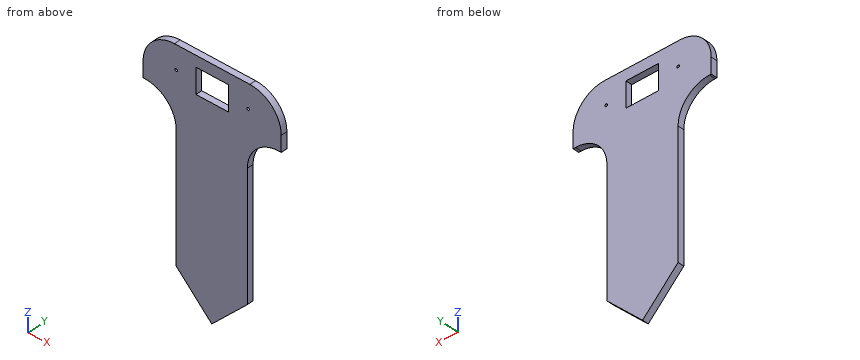
from build123d import *

# Parameters (mm, degrees)
SKETCH2_W               = 44
SKETCH2_H               = 15
BOSS_EXTRUDE1_DEPTH     = 2
SKETCH3_W               = 10.3
SKETCH3_H               = 8
CUT_EXTRUDE1_DEPTH      = 2
SKETCH5_R               = 0.4
CUT_EXTRUDE2_DEPTH      = 2
SKETCH6_W               = 22.666596939
SKETCH6_H               = 61.385041888
BOSS_EXTRUDE3_DEPTH     = 2
FILLET1_R               = 10
CUT_EXTRUDE3_DEPTH      = 73.340507297
CUT_EXTRUDE3_DEPTH_BACK = 2
CUT_EXTRUDE4_DEPTH      = 73.340507297
CUT_EXTRUDE4_DEPTH_BACK = 2
FILLET2_R               = 10


with BuildPart() as part:
    # Sketch2 → Boss-Extrude1 (new body)
    with BuildSketch(Plane(origin=(0, 0, 0), x_dir=(1, 0, 0), z_dir=(0, 1, 0))):
        Rectangle(SKETCH2_W, SKETCH2_H)
    extrude(amount=BOSS_EXTRUDE1_DEPTH)

    # Sketch3 → Cut-Extrude1 (cut)
    with BuildSketch(Plane(origin=(0, 2, 0), x_dir=(1, 0, 0), z_dir=(0, 1, 0))):
        Rectangle(SKETCH3_W, SKETCH3_H)
    extrude(amount=-CUT_EXTRUDE1_DEPTH, mode=Mode.SUBTRACT)

    # Sketch5 → Cut-Extrude2 (cut)
    with BuildSketch(Plane(origin=(0, 2, 0), x_dir=(1, 0, 0), z_dir=(0, 1, 0))):
        with Locations(Location((-11.45, 0, 0), (0, 0, 270))):
            Circle(SKETCH5_R)
    cut_extrude2 = extrude(amount=-CUT_EXTRUDE2_DEPTH, mode=Mode.SUBTRACT)

    # Mirror1: Cut-Extrude2 across plane
    add(cut_extrude2.mirror(Plane(origin=(0, 0, 0), x_dir=(0, 0, 1), z_dir=(1, 0, 0))), mode=Mode.SUBTRACT)

    # Sketch6 → Boss-Extrude3 (add)
    with BuildSketch(Plane(origin=(0, 2, 0), x_dir=(1, 0, 0), z_dir=(0, 1, 0))):
        with Locations((-0.116701531, 38.192520944)):
            Rectangle(SKETCH6_W, SKETCH6_H)
    extrude(amount=-BOSS_EXTRUDE3_DEPTH)

    # Fillet1
    fillet1_edges = [part.edges().sort_by_distance(p)[0] for p in [
        (-11.45, 1, -7.5),
        (11.216596939, 1, -7.5),
    ]]
    fillet(fillet1_edges, radius=FILLET1_R)

    # Sketch8 → Cut-Extrude3 (cut, two sides: drawn at the far end of the back side and taken through both)
    with BuildSketch(Plane(origin=(0, 2, 0), x_dir=(1, 0, 0), z_dir=(0, 1, 0)).offset(-CUT_EXTRUDE3_DEPTH_BACK)):
        Polygon((119.416120766, 188.417864185), (-0.11670153, 68.885041888), (-11.45, 57.551743419), (-130.982822296, -61.981078878), (-370.048466889, 177.084565715), (-119.649523827, 427.483508777), align=None)
    extrude(amount=CUT_EXTRUDE3_DEPTH + CUT_EXTRUDE3_DEPTH_BACK, mode=Mode.SUBTRACT)

    # Sketch9 → Cut-Extrude4 (cut, two sides: drawn at the far end of the back side and taken through both)
    with BuildSketch(Plane(origin=(0, 2, 0), x_dir=(1, 0, 0), z_dir=(0, 1, 0)).offset(-CUT_EXTRUDE4_DEPTH_BACK)):
        Polygon((-119.649523827, 188.417864185), (-0.11670153, 68.885041888), (11.216596939, 57.551743419), (130.749419236, -61.981078878), (369.815063828, 177.084565715), (119.416120766, 427.483508777), align=None)
    extrude(amount=CUT_EXTRUDE4_DEPTH + CUT_EXTRUDE4_DEPTH_BACK, mode=Mode.SUBTRACT)

    # Fillet2
    fillet2_edges = [part.edges().sort_by_distance(p)[0] for p in [
        (22, 1, 7.5),
        (-22, 1, 7.5),
    ]]
    fillet(fillet2_edges, radius=FILLET2_R)


solid = part.part
Build history of the part. All positions in model axes, mm. Round coordinates to 2 decimals unless told otherwise and drop trailing zeros. Write each loop counter-clockwise with the first axis right and the second up, starting at its lowest first coordinate (ties: lowest second). Pieces come first, ordered by that corner, then holes. Notation, with made-up numbers: (-26.75, 49) -> (25.25, 49) arc R30 cw to (25.25, 84) -> close; hole circle Ø2 at (44, 14). An arc over 180 degrees is marked (long way). Use one line per item in the form item = value.
Q1. Drill centre lines: L1, parallel to X at y = 1.2, z = -42.5; L2, parallel to X at y = 0.4, z = 0; L3, parallel to Z at x = -4.5, y = 1.25. Where is each one in solid material? Low to high.
Conclusion:
L1 = -11.45 to 11.22
L2 = -21.68 to -11.85, -11.05 to -5.15, 5.15 to 11.05, 11.85 to 21.68
L3 = -64.5 to -4, 4 to 7.5
Q2. Band-saw the part on C-C, the plane x = 1.5. Write the cut outline in (y, z), then the cut area to 3 significant figures.
Conclusion:
outline = (0, -67.27) -> (2, -67.27) -> (2, -4) -> (0, -4) -> close; (0, 4) -> (2, 4) -> (2, 7.5) -> (0, 7.5) -> close
area = 134 mm²
Q3. Band-saw the part on D-D, the plane z = -60. Write the cut outline in (x, y), then the cut area to 3 significant figures.
Conclusion:
outline = (-9, 0) -> (8.77, 0) -> (8.77, 2) -> (-9, 2) -> close
area = 35.5 mm²
Q4. Drop flat-ended pins along their axis: P1, Ø0.6, axis at y = 1, z = -46.5, coming from the -X side; P2, Ø0.6, axis at x = -2.5, y = 1.5, coming from the -Z side; P3, Ø0.6, axis at y = 1, z = -43, coming from the +X side. Give the stop position or say it passes through.
Conclusion:
P1 = -11.45
P2 = -66.8
P3 = 11.22
Q5. Band-saw the part on A-A, the plane x = -4. Write the cut outline in (y, z), then the cut area to 3 significant figures.
Conclusion:
outline = (0, -65) -> (2, -65) -> (2, -4) -> (0, -4) -> close; (0, 4) -> (2, 4) -> (2, 7.5) -> (0, 7.5) -> close
area = 129 mm²
Q6. Band-saw the part on B-B, the plane z = -41.5. Write the cut outline in (x, y), then the cut area to 3 significant figures.
Conclusion:
outline = (-11.45, 0) -> (11.22, 0) -> (11.22, 2) -> (-11.45, 2) -> close
area = 45.3 mm²
